```python
from build123d import *

# Parameters (mm, degrees)
F0_W         = 304.8
F0_H         = 215.9
F1_DEPTH     = 6.35
F2_R         = 5.08
F3_T1_DEPTH  = 13.97
F3_S5_W      = 5.08
F3_S5_H      = 5.08
F3_T6_DEPTH  = 5.08
F3_S11_W     = 5.08
F3_S11_H     = 5.08
F3_T12_DEPTH = 5.08
F3_S17_W     = 5.08
F3_S17_H     = 5.08
F3_T18_DEPTH = 5.08


# Not quite as in the source:
# - a fillet or chamfer that OpenCascade refuses, or shapes differently, is made with other operations: its cross-section is extruded or revolved along the edge and cut away or added


with BuildPart() as f1:
    # F0 (on Top) → F1 (new body)
    with BuildSketch(Plane.XY):
        with Locations((0.3756433725, 24.0940256725)):
            Rectangle(F0_W, F0_H)
    extrude(amount=F1_DEPTH)

    # F2
    f2_edges = [f1.edges().sort_by_distance(p)[0] for p in [
        (152.775643, -83.855974, 3.175),
        (0.375643, -83.855974, 6.35),
        (-152.024357, 24.094026, 6.35),
        (0.375643, 132.044026, 6.35),
        (152.775643, 24.094026, 6.35),
    ]]
    fillet(f2_edges, radius=F2_R)

    # F3: fillet of radius 5.08 on 3 edges, made by hand

    # F3_s2 → F3_t1 (cut)
    with BuildSketch(Plane.XY.offset(-12.7)):
        with BuildLine():
            ThreePointArc((-152.0243566275, -78.7759743275), (-150.5364590759, -82.3680767759), (-146.9443566275, -83.8559743275))
            Line((-146.9443566275, -83.8559743275), (-152.0243566275, -83.8559743275))
            Line((-152.0243566275, -83.8559743275), (-152.0243566275, -78.7759743275))
        make_face()
        with BuildLine():
            ThreePointArc((-146.9443566275, 132.0440256725), (-150.5364590759, 130.556128121), (-152.0243566275, 126.9640256725))
            Line((-152.0243566275, 126.9640256725), (-152.0243566275, 132.0440256725))
            Line((-152.0243566275, 132.0440256725), (-146.9443566275, 132.0440256725))
        make_face()
        with BuildLine():
            ThreePointArc((152.7756433725, 126.9640256725), (151.287745821, 130.556128121), (147.6956433725, 132.0440256725))
            Line((147.6956433725, 132.0440256725), (152.7756433725, 132.0440256725))
            Line((152.7756433725, 132.0440256725), (152.7756433725, 126.9640256725))
        make_face()
    extrude(amount=F3_T1_DEPTH, mode=Mode.SUBTRACT)


with BuildPart() as f3_tool4:
    # F3_s5 → F3_t6 (new body)
    with BuildSketch(Plane.YZ.offset(147.6956433725)):
        with Locations((129.5040256725, 3.81)):
            Rectangle(F3_S5_W, F3_S5_H)
    extrude(amount=F3_T6_DEPTH)

    # F3_s7 → F3_t8 (revolve, cut)
    with BuildSketch(Plane(origin=(147.6956433725, 126.9640256725, 1.27), x_dir=(0, -0.7071067812, -0.7071067812), z_dir=(0, -0.7071067812, 0.7071067812))):
        with BuildLine():
            ThreePointArc((0, -5.08), (5.08, 0), (0, 5.08))
            Line((0, 5.08), (0, -5.08))
        make_face()
    revolve(axis=Axis((147.6956433725, 126.9640256725, 1.27), (1, 0, 0)), mode=Mode.SUBTRACT)


with BuildPart() as f1_1:
    add(f1.part)

    # F3_t3: cut F3_tool4
    add(f3_tool4.part, mode=Mode.SUBTRACT)


with BuildPart() as f3_tool10:
    # F3_s11 → F3_t12 (new body)
    with BuildSketch(Plane.XZ.offset(-126.9640256725)):
        with Locations((-149.4843566275, 3.81)):
            Rectangle(F3_S11_W, F3_S11_H)
    extrude(amount=-F3_T12_DEPTH)

    # F3_s13 → F3_t14 (revolve, cut)
    with BuildSketch(Plane(origin=(-146.9443566275, 126.9640256725, 1.27), x_dir=(0.7071067812, 0, -0.7071067812), z_dir=(0.7071067812, 0, 0.7071067812))):
        with BuildLine():
            ThreePointArc((0, -5.08), (5.08, 0), (0, 5.08))
            Line((0, 5.08), (0, -5.08))
        make_face()
    revolve(axis=Axis((-146.9443566275, 126.9640256725, 1.27), (0, 1, 0)), mode=Mode.SUBTRACT)


with BuildPart() as f1_2:
    add(f1_1.part)

    # F3_t9: cut F3_tool10
    add(f3_tool10.part, mode=Mode.SUBTRACT)


with BuildPart() as f3_tool16:
    # F3_s17 → F3_t18 (new body)
    with BuildSketch(Plane.YZ.offset(-146.9443566275)):
        with Locations((-81.3159743275, 3.81)):
            Rectangle(F3_S17_W, F3_S17_H)
    extrude(amount=-F3_T18_DEPTH)

    # F3_s19 → F3_t20 (revolve, cut)
    with BuildSketch(Plane(origin=(-146.9443566275, -78.7759743275, 1.27), x_dir=(0, 0.7071067812, -0.7071067812), z_dir=(0, 0.7071067812, 0.7071067812))):
        with BuildLine():
            ThreePointArc((0, -5.08), (5.08, 0), (0, 5.08))
            Line((0, 5.08), (0, -5.08))
        make_face()
    revolve(axis=Axis((-146.9443566275, -78.7759743275, 1.27), (-1, 0, 0)), mode=Mode.SUBTRACT)


with BuildPart() as f1_3:
    add(f1_2.part)

    # F3_t15: cut F3_tool16
    add(f3_tool16.part, mode=Mode.SUBTRACT)


solid = f1_3.part
```
Check sheet for the modelled part. Datum: model origin and axes. Units: mm. Round coordinates to 2 decimals unless told otherwise and drop trailing zeros. Loops run counter-clockwise (first coordinate to the right, second up) from the corner with the lowest first, then second, coordinate; pieces in that order, holes last. Notation, with made-up numbers: (29.5, 13.25) - (42.5, 13.25) arc R17 cw to (42.5, 23.25) - close; hole circle Ø2 at (11.5, -1.75). An arc over 180 degrees is marked (long way). Answer as a JSON object with one key per item and string values. Group by question number.
Q1. Scan lines: line 1 along Y through (x, z) = (127.5, 1.75); line 2 along Y through (x, z) = (118.5, 1.5); line 3 along X through (y, z) = (31, 2.5). Record each from-to range of solid material in increasing order. Write a range as [from, to].
Q2. Sectioned sample at A-A, the plane z = 4.75. Enter the section's corners in (x, y), plus the area to 3 significant figures.
Q3. Gauge pin test, flat end, axial feed: P1, Ø1.5, axis at y = 108, z = 5, coming from the +X side. Record the tip position at first contact, or that the pin passes through.
Solution:
{
 "1": {"line 1": "y = [-83.83, 132.02]", "line 2": "y = [-83.85, 132.04]", "line 3": "x = [-151.87, 152.62]"},
 "2": {"outline": "(-150.65, -78.78) arc R3.7 ccw to (-146.94, -82.48) - (147.7, -82.48) arc R3.7 ccw to (151.4, -78.78) - (151.4, 126.96) arc R3.7 ccw to (147.7, 130.66) - (-146.94, 130.66) arc R3.7 ccw to (-150.65, 126.96) - close", "area": "64,400 mm²"},
 "3": {"P1": "stops at x = 151.81"}
}
